```python
from build123d import *

# Parameters (mm, degrees)
SKETCH1_R           = 4
SKETCH1_W           = 3.5
SKETCH1_H           = 5.5
SKETCH1_W_2         = 15
SKETCH1_H_2         = 3
BOSS_EXTRUDE1_DEPTH = 3


with BuildPart() as part:
    # Sketch1 → Boss-Extrude1 (new body)
    with BuildSketch(Plane(origin=(0, 0, 0), x_dir=(1, 0, 0), z_dir=(0, 1, 0))):
        with BuildLine():
            Line((0, 0), (-25, 0))
            Line((-25, 0), (-25, -47.5))
            ThreePointArc((-25, -47.5), (-12.5, -60), (0, -47.5))
            Line((0, -47.5), (0, 0))
        make_face()
        with Locations(Location((-12.5, -15, 0), (0, 0, 270))):
            Circle(SKETCH1_R, mode=Mode.SUBTRACT)
        with Locations((-21, -5)):
            Rectangle(SKETCH1_W, SKETCH1_H, mode=Mode.SUBTRACT)
        with Locations((-4, -5)):
            Rectangle(SKETCH1_W, SKETCH1_H, mode=Mode.SUBTRACT)
        with Locations((-21, -20)):
            Rectangle(SKETCH1_W, SKETCH1_H, mode=Mode.SUBTRACT)
        with Locations((-4, -20)):
            Rectangle(SKETCH1_W, SKETCH1_H, mode=Mode.SUBTRACT)
        with Locations((-12.5, -48.75)):
            Rectangle(SKETCH1_W_2, SKETCH1_H_2, mode=Mode.SUBTRACT)
    extrude(amount=BOSS_EXTRUDE1_DEPTH)


solid = part.part
```
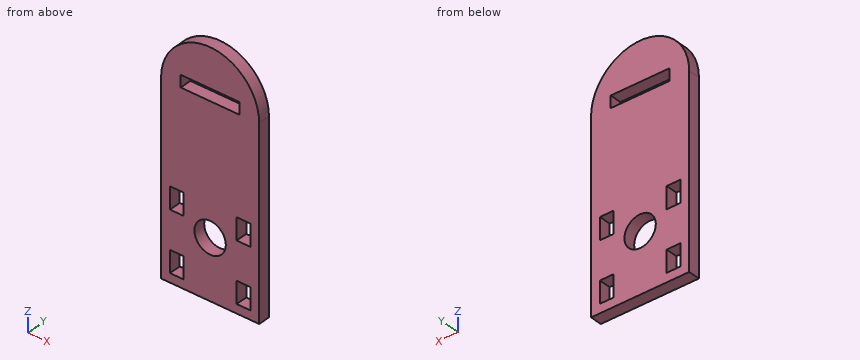
Work out the finished part from the listing and answer in its coordinate system (mm). Give positions to 0.01 mm unless a question says otherwise; leave off trailing zeros. Loops run counter-clockwise (first coordinate to the right, second up) from the corner with the lowest first, then second, coordinate; pieces in that order, holes last. Notation, with made-up numbers: (36.25, 43.25) -> (78.25, 43.25) arc R9 cw to (78.25, 49.25) -> close; hole circle Ø8 at (69.25, 18). An arc over 180 degrees is marked (long way). Use CSV: the item, a comma, the result in double quotes.
1. Straight lines are drawn through the part: line 1 (X direction, y = 0.9, z = 7.5); line 2 (Z direction, x = -9, y = 2.8); line 3 (Z direction, x = -10.5, y = 1.5). For each, find the intervals that lie inside material, in ascending order.
Found:
line 1,"-25 to -22.75, -19.25 to -5.75, -2.25 to 0"
line 2,"0 to 13.06, 16.94 to 47.25, 50.25 to 59.5"
line 3,"0 to 11.54, 18.46 to 47.25, 50.25 to 59.84"
2. The part is cut by section D-D (x = -7). Write down the section's boundary in (y, z).
Found:
outline,"(0, 0) -> (3, 0) -> (3, 47.25) -> (0, 47.25) -> close; (0, 50.25) -> (3, 50.25) -> (3, 58.72) -> (0, 58.72) -> close"
3. The part is cut by section A-A (z = 15). Write down the section's boundary in (x, y).
Found:
outline,"(-25, 0) -> (-16.5, 0) -> (-16.5, 3) -> (-25, 3) -> close; (-8.5, 0) -> (0, 0) -> (0, 3) -> (-8.5, 3) -> close"
4. The part is cut by section B-B (x = -12.5). Write down the section's boundary in (y, z), then the cut area to 3 significant figures.
Found:
outline,"(0, 0) -> (3, 0) -> (3, 11) -> (0, 11) -> close; (0, 19) -> (3, 19) -> (3, 47.25) -> (0, 47.25) -> close; (0, 50.25) -> (3, 50.25) -> (3, 60) -> (0, 60) -> close"
area,"147 mm^2"
5. The part is cut by section C-C (y = 0.6). Write down the section's boundary in (x, z), then the cut area to 3 significant figures.
Found:
outline,"(-25, 0) -> (0, 0) -> (0, 47.5) arc R12.5 ccw to (-25, 47.5) -> close; hole (-22.75, 2.25) -> (-19.25, 2.25) -> (-19.25, 7.75) -> (-22.75, 7.75) -> close; hole (-22.75, 17.25) -> (-19.25, 17.25) -> (-19.25, 22.75) -> (-22.75, 22.75) -> close; hole (-20, 47.25) -> (-5, 47.25) -> (-5, 50.25) -> (-20, 50.25) -> close; hole circle Ø8 at (-12.5, 15); hole (-5.75, 2.25) -> (-2.25, 2.25) -> (-2.25, 7.75) -> (-5.75, 7.75) -> close; hole (-5.75, 17.25) -> (-2.25, 17.25) -> (-2.25, 22.75) -> (-5.75, 22.75) -> close"
area,"1,260 mm^2"
6. Flat-ended cylindrical pins translate along their axes: pin 1 Ø0.9 at (x, y) = (-4, 1) entering from +Z; pin 2 Ø1.5 at (y, z) = (2, 4.5) entering from +X; pin 3 Ø1 at (x, y) = (-7, 2.5) entering from +Z; pin 4 Ø5 at (x, z) = (-12.5, 15) entering from -Y. Find the tip coordinate at first contact, or state that the pin passes through.
Found:
pin 1,"z = 57.06"
pin 2,"x = 0"
pin 3,"z = 58.96"
pin 4,"through"
